CAD build for the part. Positions are in the model's coordinates, mm. Round coordinates to 2 decimals unless told otherwise and drop trailing zeros. Order: outer loops, then holes, each group sorted by start corner. A loop starts at its lowest first (then second) coordinate and runs counter-clockwise, first axis right, second up. Notation, with made-up numbers: (53, 17) - (76, 17) arc R23 cw to (76, 48) - close; hole circle Ø9 at (65.25, -6). An arc over 180 degrees is marked (long way). Use one line per item in the form item = value. Start each with the question number.
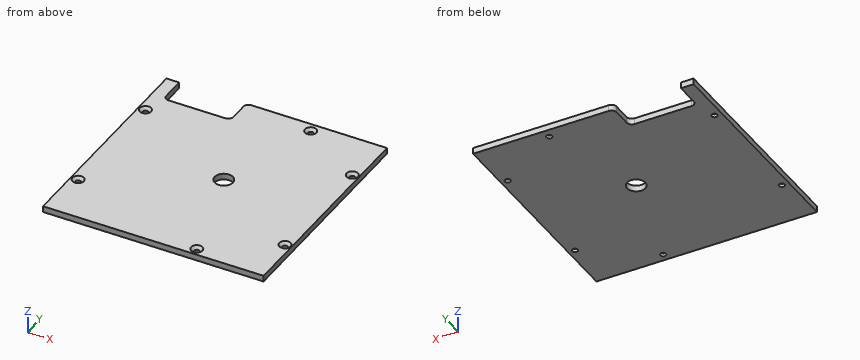
from build123d import *

# Parameters (mm, degrees)
ESBO_O1_W                            = 217
ESBO_O1_H                            = 220
RESSALTO_EXTRUS_O1_DEPTH             = 6
ESCAREADO_PARA_SFHCS_M51_D           = 5.5
ESCAREADO_PARA_SFHCS_M51_CSINK_D     = 11.2
ESCAREADO_PARA_SFHCS_M51_CSINK_ANGLE = 90
CORTE_EXTRUS_O1_REACH                = 162.702
ESBO_O5_R                            = 9
ESBO_O6_W                            = 66
ESBO_O6_H                            = 28
CORTE_EXTRUS_O2_DEPTH                = 161.7015868
FILETE1_R                            = 5


with BuildPart() as part:
    # Esboço1 → Ressalto-extrusão1 (new body)
    with BuildSketch(Plane.XY):
        with Locations((-8.5, 0)):
            Rectangle(ESBO_O1_W, ESBO_O1_H)
    extrude(amount=RESSALTO_EXTRUS_O1_DEPTH)

    # Escareado para SFHCS M51 (through all)
    with Locations(Plane.XY.offset(6)):
        with Locations((-110, -60), (-110, 60), (93.5, 60), (93.5, -60), (30, -102.194888391), (30, 100.827560784)):
            CounterSinkHole(ESCAREADO_PARA_SFHCS_M51_D / 2, ESCAREADO_PARA_SFHCS_M51_CSINK_D / 2, counter_sink_angle=ESCAREADO_PARA_SFHCS_M51_CSINK_ANGLE)

    # Esboço5 → Corte-extrusão1 (cut, up to next)
    with BuildSketch(Plane.XY.offset(6), mode=Mode.PRIVATE) as corte_extrus_o1_sk1:
        with Locations((0, 0.3)):
            Circle(ESBO_O5_R)
    corte_extrus_o1_tool1 = extrude(corte_extrus_o1_sk1.sketch, amount=-CORTE_EXTRUS_O1_REACH, mode=Mode.PRIVATE) & part.part
    add(corte_extrus_o1_tool1.solids().sort_by_distance((0, 0.3, 6))[0], mode=Mode.SUBTRACT)

    # Esboço6 → Corte-extrusão2 (cut, through all)
    with BuildSketch(Plane.XY.offset(6)):
        with Locations((-71.5, 96)):
            Rectangle(ESBO_O6_W, ESBO_O6_H)
    extrude(amount=-CORTE_EXTRUS_O2_DEPTH, mode=Mode.SUBTRACT)

    # Filete1
    filete1_edges = [part.edges().sort_by_distance(p)[0] for p in [
        (-104.5, 82, 3),
        (-38.5, 110, 3),
        (-38.5, 82, 3),
    ]]
    fillet(filete1_edges, radius=FILETE1_R)


solid = part.part
(1) Flat gauge pin, fed straight in: P1, Ø6.5, axis at x = 30, y = 100.83, coming from the +Z side. Where does the tip first touch, or does it go through?
(2) Slice it at B-B (y = 60). Give the cut face in (x, z), and give its area (3 significant figures).
(3) Slice it at C-C (x = 0). Give the cut face in (y, z).
(4) Slice it at D-D (z = 1.9). Give the cut face in (x, y).
(5) Slice it at A-A (x = 30). Give the cut face in (y, z).
(6) Wall check: line 1 (X direction, y = 60, z = 0.9); line 2 (Y direction, x = 30, z = 0.9); line 3 (Y direction, x = -110, z = 2.15). Give the ranges that are in metal, low to high. Write a range as [from, to].
Results list:
q1.P1 = 3.65
q2.outline = (-117, 0) - (-112.75, 0) - (-112.75, 3.15) - (-115.6, 6) - (-117, 6) - close; (-107.25, 0) - (90.75, 0) - (90.75, 3.15) - (87.9, 6) - (-104.4, 6) - (-107.25, 3.15) - close; (96.25, 0) - (100, 0) - (100, 6) - (99.1, 6) - (96.25, 3.15) - close
q2.area = 1,220 mm²
q3.outline = (-110, 0) - (-8.7, 0) - (-8.7, 6) - (-110, 6) - close; (9.3, 0) - (110, 0) - (110, 6) - (9.3, 6) - close
q4.outline = (-117, -110) - (100, -110) - (100, 110) - (-33.5, 110) arc R5 ccw to (-38.5, 105) - (-38.5, 87) arc R5 cw to (-43.5, 82) - (-99.5, 82) arc R5 cw to (-104.5, 87) - (-104.5, 110) - (-117, 110) - close; hole circle Ø5.5 at (-110, -60); hole circle Ø5.5 at (-110, 60); hole circle Ø18 at (0, 0.3); hole circle Ø5.5 at (30, -102.19); hole circle Ø5.5 at (30, 100.83); hole circle Ø5.5 at (93.5, -60); hole circle Ø5.5 at (93.5, 60)
q5.outline = (-110, 0) - (-104.94, 0) - (-104.94, 3.15) - (-107.79, 6) - (-110, 6) - close; (-99.44, 0) - (98.08, 0) - (98.08, 3.15) - (95.23, 6) - (-96.59, 6) - (-99.44, 3.15) - close; (103.58, 0) - (110, 0) - (110, 6) - (106.43, 6) - (103.58, 3.15) - close
q6.line_1 = [-117, -112.75], [-107.25, 90.75], [96.25, 100]
q6.line_2 = [-110, -104.94], [-99.44, 98.08], [103.58, 110]
q6.line_3 = [-110, -62.75], [-57.25, 57.25], [62.75, 110]
